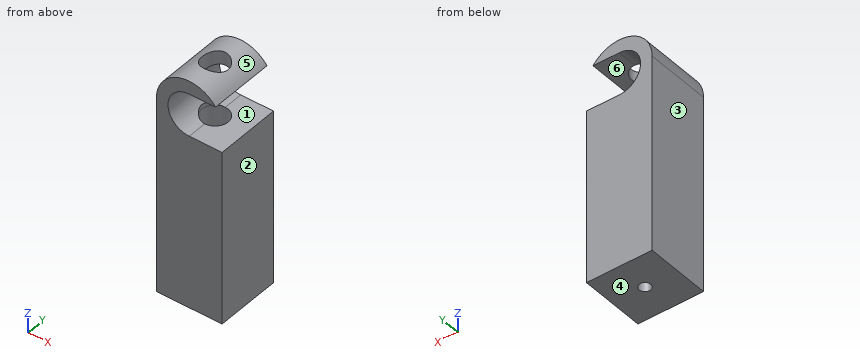
```python
from build123d import *

# Parameters (mm, degrees)
F1_DEPTH      = 10
F1_DEPTH_BACK = 10
F3_DEPTH      = 20
F4_R          = 4
F5_DEPTH      = 40
F5_DEPTH_BACK = 18.0000001001
F7_D          = 3.5


with BuildPart() as f1:
    # F0 (on Front) → F1 (new body, two sides)
    with BuildSketch(Plane.XZ) as f1_sk:
        with BuildLine():
            ThreePointArc((10, 60), (0, 70), (-10, 60))
            Line((-10, 60), (-10, 0))
            Line((-10, 0), (10, 0))
            Line((10, 0), (10, 60))
        make_face()
    extrude(amount=F1_DEPTH)
    extrude(f1_sk.sketch, amount=-F1_DEPTH_BACK)

    # F2 (on face) → F3 (cut, through all)
    with BuildSketch(Plane(origin=(0, 10, 0), x_dir=(-1, 0, 0), z_dir=(0, 1, 0))):
        with BuildLine():
            Line((-10, 53), (0, 53))
            ThreePointArc((0, 53), (6.5, 59.5), (0, 66))
            Line((0, 66), (-8, 66))
            ThreePointArc((-8, 66), (-9.4868329805, 63.1622776602), (-10, 60))
            Line((-10, 60), (-10, 53))
        make_face()
    extrude(amount=-F3_DEPTH, mode=Mode.SUBTRACT)

    # F4 (on face) → F5 (cut, two sides)
    with BuildSketch(Plane.XY.offset(53)) as f5_sk:
        Circle(F4_R)
    extrude(amount=-F5_DEPTH, mode=Mode.SUBTRACT)
    extrude(f5_sk.sketch, amount=F5_DEPTH_BACK, mode=Mode.SUBTRACT)

    # F7 (through all)
    with Locations(Plane.XY.offset(13)):
        with Locations((0, 0)):
            Hole(F7_D / 2)


solid = f1.part
```
Source: CAD feature listing. Evaluate the final solid. Frame: model axes, mm. Face numbers are marked on the shaded views. A direction names the side the tool comes from. Round coordinates to 2 decimals unless told otherwise and drop trailing zeros. Order: outer loops, then holes, each group sorted by start corner. A loop starts at its lowest first (then second) coordinate and runs counter-clockwise, first axis right, second up. Notation, with made-up numbers: (2, 41) -> (58, 41) arc R23 ccw to (58, 63) -> close; hole circle Ø11 at (73.5, 25.25). An arc over 180 degrees is marked (long way). Use CSV: the item, a comma, the result in double quotes.
(1) Section C-C on z = 50. Return the cut outline in (x, y).
Report:
outline,"(-10, -10) -> (10, -10) -> (10, 10) -> (-10, 10) -> close; hole circle Ø8 at (0, 0)"
(2) Section A-A on y = -2.75. Return the cut outline in (x, z), and give its area (3 significant figures).
Report:
outline,"(-10, 0) -> (10, 0) -> (10, 53) -> (2.9, 53) -> (2.9, 13) -> (-2.9, 13) -> (-2.9, 53.69) arc R6.5 cw to (-2.9, 65.31) -> (-2.9, 69.57) arc R10 ccw to (-10, 60) -> close; (2.9, 66) -> (8, 66) arc R10 ccw to (2.9, 69.57) -> close"
area,"908 mm^2"
(3) Access query for the marked faces 1 and 2. Directions: +Z, -Z, +X, -X, +Y, -Y. A direction counts if a zero-diameter tool reaches every point of the face in a straight line with its end or side. Return the directions, or none.
Report:
face 1,"+X, +Y, -Y"
face 2,"+Z, -Z, +X, +Y, -Y"
(4) Ray query, L1, parallel to Y at x = 0, z = 29; L2, parallel to Y at x = 0, z = 4.5. Return the intervals inside material, ascending.
Report:
L1,"-10 to -4, 4 to 10"
L2,"-10 to -1.75, 1.75 to 10"
(5) Section D-D on x = -8.5. Return the cut outline in (y, z).
Report:
outline,"(-10, 0) -> (10, 0) -> (10, 65.27) -> (-10, 65.27) -> close"
(6) First-contact query: pin 1 Ø5.5 at (x, y) = (0, 0) entering from +Z; pin 2 Ø2 at (x, y) = (-8, 1.5) entering from +Z. Flat tips, straight axial feed; report the tip coordinate or a pass-through.
Report:
pin 1,"z = 13"
pin 2,"z = 67.14"
(7) Section B-B on y = 0. Return the cut outline in (x, z).
Report:
outline,"(-10, 0) -> (-1.75, 0) -> (-1.75, 13) -> (-4, 13) -> (-4, 54.38) arc R6.5 cw to (-4, 64.62) -> (-4, 69.17) arc R10 ccw to (-10, 60) -> close; (1.75, 0) -> (10, 0) -> (10, 53) -> (4, 53) -> (4, 13) -> (1.75, 13) -> close; (4, 66) -> (8, 66) arc R10 ccw to (4, 69.17) -> close"
(8) Pull-direction query (Z, two-part tool) for the marked faces 3, 4, 5 and 6; classes: +Z half, -Z half, draft (parallel to the pull), parting line (faces both ways), or undercut.
Report:
face 3,"draft"
face 4,"-Z half"
face 5,"+Z half"
face 6,"undercut"
